CAD build for the part. Positions are in the model's coordinates, mm. Face numbers are marked on the shaded views. A direction names the side the tool comes from. Give positions to 0.01 mm unless a question says otherwise; leave off trailing zeros. Loops run counter-clockwise (first coordinate to the right, second up) from the corner with the lowest first, then second, coordinate; pieces in that order, holes last. Notation, with made-up numbers: M 63.25,47 L 97.25,47 A19 ccw 97.25,81 Z; hole C -10,-16 d7. An arc over 180 degrees is marked long. Answer as CSV lines item,"result".
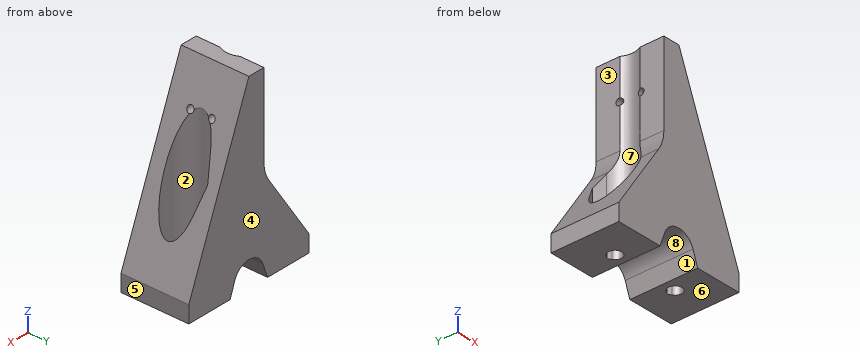
```python
from build123d import *

# Parameters (mm, degrees)
BOSS_EXTRUDE1_DEPTH   = 12.7
CUT_EXTRUDE1_DEPTH    = 10.525
CUT_EXTRUDE2_DEPTH    = 61.3250001
LPATTERN1_COUNT       = 2
LPATTERN1_PITCH       = 25.4
M3X0_5_TAPPED_HOLE1_D = 2.5


with BuildPart() as part:
    # Sketch1 → Boss-Extrude1 (new body, symmetric)
    with BuildSketch(Plane(origin=(0, 0, 0), x_dir=(1, 0, 0), z_dir=(0, 1, 0))):
        with BuildLine():
            Line((0, 0), (17.4625, 0))
            Line((17.4625, 0), (19.441706855, -5.370732862))
            ThreePointArc((19.441706855, -5.370732862), (25.4, -9.525), (31.358293145, -5.370732862))
            Line((31.358293145, -5.370732862), (33.3375, 0))
            Line((33.3375, 0), (50.8, 0))
            Line((50.8, 0), (50.8, -6.35))
            Line((50.8, -6.35), (25.4, -69.85))
            Line((25.4, -69.85), (19.05, -69.85))
            Line((19.05, -69.85), (19.05, -38.770250599))
            ThreePointArc((19.05, -38.770250599), (18.505068736, -35.089991911), (16.917038738, -31.725558107))
            Line((16.917038738, -31.725558107), (0, -6.35))
            Line((0, -6.35), (0, 0))
        make_face()
    extrude(amount=BOSS_EXTRUDE1_DEPTH, both=True)

    # Sketch2 → Cut-Revolve1 (revolve, cut)
    with BuildSketch(Plane(origin=(0, 0, 0), x_dir=(1, 0, 0), z_dir=(0, 1, 0))):
        Polygon((12.7, 0), (12.7, -120.015), (5.334, -120.015), (5.334, -9.525), (10.1473, -9.525), (10.1473, 0), align=None)
    cut_revolve1 = revolve(axis=Axis((12.7, 0, 0), (0, 0, -1)), mode=Mode.SUBTRACT)

    # Sketch6 → Cut-Extrude1 (cut, through all)
    with BuildSketch(Plane.XY.offset(9.525)):
        with BuildLine():
            Line((11.42365, 2.210703048), (12.7, 2.947604064))
            Line((12.7, 2.947604064), (13.97635, 2.210703048))
            ThreePointArc((13.97635, 2.210703048), (12.7, 2.5527), (11.42365, 2.210703048))
        make_face()
    cut_extrude1 = extrude(amount=-CUT_EXTRUDE1_DEPTH, mode=Mode.SUBTRACT)

    # Sketch7 → Cut-Extrude2 (cut, through all)
    with BuildSketch(Plane.XY.offset(9.525)):
        with BuildLine():
            Line((9.017, 6.379143124), (12.7, 8.505524166))
            Line((12.7, 8.505524166), (16.383, 6.379143124))
            ThreePointArc((16.383, 6.379143124), (12.7, 7.366), (9.017, 6.379143124))
        make_face()
    cut_extrude2 = extrude(amount=CUT_EXTRUDE2_DEPTH, mode=Mode.SUBTRACT)

    # LPattern1: Cut-Revolve1, Cut-Extrude1, Cut-Extrude2 ×2
    with Locations(*[(i * LPATTERN1_PITCH, 0, 0) for i in range(1, LPATTERN1_COUNT)]):
        add(cut_revolve1, mode=Mode.SUBTRACT)
        add(cut_extrude1, mode=Mode.SUBTRACT)
        add(cut_extrude2, mode=Mode.SUBTRACT)

    # M3x0.5 Tapped Hole1 (through all)
    with Locations(Plane.ZY.offset(-19.05)):
        with Locations((55, 4), (55, -4)):
            Hole(M3X0_5_TAPPED_HOLE1_D / 2)


solid = part.part
```
Q1. Wall check: line 1 (Y direction, x = 26, z = 55); line 2 (Y direction, x = 38.1, z = 3); line 3 (X direction, y = 0, z = 29). Give the ranges that are in metal, low to high. Write a range as [from, to].
Solution:
line 1,"y = [-12.7, -5.25], [-2.75, 2.75], [5.25, 12.7]"
line 2,"y = [-12.7, -2.55], [2.95, 12.7]"
line 3,"x = [20.07, 30.73]"
Q2. Cut at A-A (y = 0). Give the number of separate pieces and of enclosed holes in the cut face, and give its area (3 significant figures).
Solution:
separate pieces,"3"
enclosed holes,"0"
area,"907 mm²"
Q3. Cut at C-C (x = 24). Write the cut outline in (y, z).
Solution:
outline,"M -12.7,9.37 L 12.7,9.37 L 12.7,69.85 L -12.7,69.85 Z; hole C -4,55 d2.5; hole C 4,55 d2.5"
Q4. Pin check, flat tips, straight feed: P1, Ø7.5, axis at x = 16, y = -0.5, coming from the +Z side (3 decimals); P2, Ø10, axis at y = 10, z = 60, coming from the -X side; P3, Ø5, axis at y = -3.5, z = 38.5, coming from the +X side. Stop position of each tip, or through.
Solution:
P1,"stops at z = 9.525"
P2,"stops at x = 19.05"
P3,"stops at x = 33.83"
Q5. Which spindle directions (+Z, -Z, +X, -X, +Y, -Y) get a long thin tool onto all of the face, cutting with end or side? Do the marked faces 1, 2, 3 and 4. Say none if no direction does.
Solution:
face 1,"-Z, +Y, -Y"
face 2,"+Z"
face 3,"+Z, -X, +Y, -Y"
face 4,"+Z, -Z, +X, -X, +Y"
Q6. Mould opens along X. For the marked faces 5, 6, 7 and 8 say: released by +X, released by -X, zero draft, split by the parting line, or undercut.
Solution:
face 5,"released by +X"
face 6,"zero draft"
face 7,"undercut"
face 8,"undercut"
Q7. Cut at B-B (z = 19). Write the cut outline in (x, y), and give its area (3 significant figures).
Solution:
outline,"M 8.43,-12.7 L 45.74,-12.7 L 45.74,12.7 L 8.43,12.7 L 8.43,6 A7.37 cw 9.02,6.38 L 12.7,8.51 L 16.38,6.38 A7.37 cw long 8.43,-6 Z; hole M 34.42,6.38 A7.37 ccw long 41.78,6.38 L 38.1,8.51 Z"
area,"627 mm²"
